Job drawing, mm, ordinate dimensions from the low corner. One solid piece. A direction names the side the tool comes from. Give positions to 0.01 mm unless a question says otherwise; leave off trailing zeros. Order: outer loops, then holes, each group sorted by start corner. A loop starts at its lowest first (then second) coordinate and runs counter-clockwise, first axis right, second up. Notation, with made-up numbers: M 1.25,52.25 L 11.25,52.25 A22 ccw 11.25,58.25 Z; hole C -26,76.5 d3. An arc over 180 degrees is marked long. Put each result on its own line as item: value. Start each with the question number.
1) Pin check, flat tips, straight feed: pin 1 (4 mm diameter, centred on x = 3, z = 7, fed in from +Y); pin 2 (1 mm diameter, centred on x = 9.5, y = 7, fed in from -Z); pin 3 (4 mm diameter, centred on y = 9, z = 5.5, fed in from -X). Stop position of each tip, or through.
2) Cut at C-C (z = 8.25). Write the cut outline in (x, y), and give its area (3 significant figures).
3) Drill centre lines: line 1 (Y direction, x = 2.5, z = 2.2) (1 decimal); line 2 (Z direction, x = 1, y = 1.75); line 3 (Y direction, x = 10, z = 1.25). Where is each one in solid material? Low to high. Write a range as [from, to].
4) Cut at B-B (z = 2). Give the number of separate pieces and of enclosed holes in the cut face, and give its area (3 significant figures).
5) Cut at D-D (y = 4.25). Write the cut outline in (x, z) (1 decimal), and give its area (3 significant figures).
6) Cut at A-A (x = 9.5). Write the cut outline in (y, z).
7) Two-plate mould, pull along X, no slides. Class the marked faces 3, 4, 5 and 6: released by +X, released by -X, zero draft, split by the parting line, or undercut.
8) Tool access for the marked faces 1 and 2: list every direction of +Z, -Z, +X, -X, +Y, -Y with a clear straight run to the whole face (end or side of a thin tool).
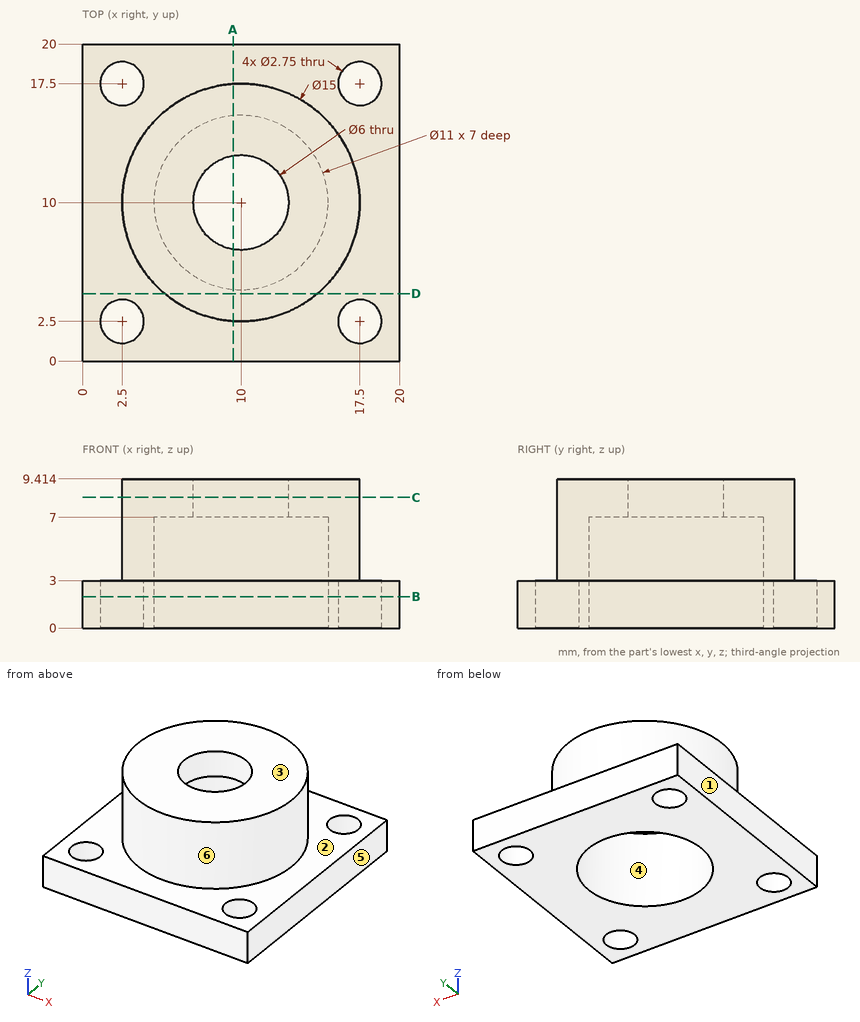
Solution:
1. pin 1: y = 15.59
1. pin 2: z = 7
1. pin 3: x = 2.5
2. outline: C 10,10 d15; hole C 10,10 d6
2. area: 148 mm²
3. line 1: [0, 1.1], [3.9, 16.1], [18.9, 20]
3. line 2: [0, 3]
3. line 3: [0, 4.5], [15.5, 20]
4. separate pieces: 1
4. enclosed holes: 5
4. area: 281 mm²
5. outline: M 0,0 L 20,0 L 20,3 L 14.8,3 L 14.8,9.4 L 5.2,9.4 L 5.2,3 L 0,3 Z
5. area: 122 mm²
6. outline: M 0,0 L 4.52,0 L 4.52,7 L 7.04,7 L 7.04,9.41 L 2.52,9.41 L 2.52,3 L 0,3 Z; M 12.96,7 L 15.48,7 L 15.48,0 L 20,0 L 20,3 L 17.48,3 L 17.48,9.41 L 12.96,9.41 Z
7. face 3: zero draft
7. face 4: undercut
7. face 5: released by +X
7. face 6: split by the parting line
8. face 1: +Z, -Z, -X, +Y, -Y
8. face 2: +Z
